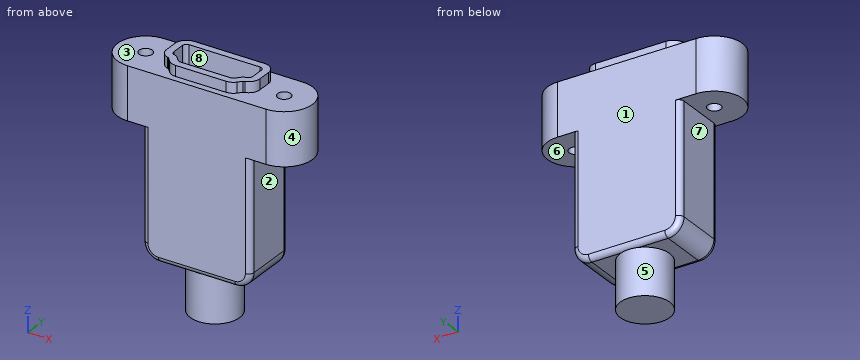
Autodesk Inventor part; units mm, degrees
ref_plane "YZ Plane" through (0, 0, 0) normal (1, 0, 0) x (0, 1, 0)
ref_plane "XZ Plane" through (0, 0, 0) normal (0, 1, 0) x (-1, 0, 0)
ref_plane "XY Plane" through (0, 0, 0) normal (0, 0, 1) x (1, 0, 0)
sketch "Sketch1" plane through (0, 0, 0) normal (0, 0, 1) x (1, 0, 0)
  line L0 (0, 0) -> (26.3, 0)
  line L1 (26.3, 10.7) -> (0, 10.7)
  arc A0 (0, 10.7) -> (0, 0) centre (0, 5.35) ccw
  arc A1 (26.3, 0) -> (26.3, 10.7) centre (26.3, 5.35) ccw
  circle A2 centre (0, 5.35) radius 1.25
  circle A3 centre (26.3, 5.35) radius 1.25
  dimension "d0" = 26.3
  dimension "d1" = 10.7
  dimension "d2" = 2.5
extrude "Extrusion1" add sketch "Sketch1" against normal blind 10
sketch "Sketch2" plane through (0, 0, 0) normal (0, 0, 1) x (1, 0, 0)
  line L0 (0, 0) -> (26.3, 0)
  arc A0 (0, 10.7) -> (0, 0) centre (0, 5.35) ccw
  line L1 (6.9455, 3.7725) -> (7.7604, 2.8465)
  line L2 (8.361, 2.575) -> (17.939, 2.575)
  line L3 (18.5396, 2.8465) -> (19.3545, 3.7725)
  line L4 (19.6057, 3.9348) -> (20.0852, 4.0824)
  line L5 (20.65, 4.847) -> (20.65, 7.325)
  line L6 (19.85, 8.125) -> (6.45, 8.125)
  line L7 (5.65, 7.325) -> (5.65, 4.847)
  line L8 (6.2148, 4.0824) -> (6.6943, 3.9348)
  line L9 (26.3, 10.7) -> (0, 10.7)
  arc A1 (6.45, 8.125) -> (5.65, 7.325) centre (6.45, 7.325) ccw
  arc A2 (20.65, 7.325) -> (19.85, 8.125) centre (19.85, 7.325) ccw
  arc A3 (5.65, 4.847) -> (6.2148, 4.0824) centre (6.45, 4.847) ccw
  arc A4 (20.0852, 4.0824) -> (20.65, 4.847) centre (19.85, 4.847) ccw
  arc A5 (6.9455, 3.7725) -> (6.6943, 3.9348) centre (6.5326, 3.4092) ccw
  arc A6 (19.6057, 3.9348) -> (19.3545, 3.7725) centre (19.7674, 3.4092) ccw
  arc A7 (7.7604, 2.8465) -> (8.361, 2.575) centre (8.361, 3.375) ccw
  arc A8 (17.939, 2.575) -> (18.5396, 2.8465) centre (17.939, 3.375) ccw
  line L10 (6.45, 9.4895) -> (19.85, 9.4895)
  arc A9 (22.0145, 7.325) -> (19.85, 9.4895) centre (19.85, 7.325) ccw
  line L11 (22.0145, 7.325) -> (22.0145, 4.847)
  arc A10 (20.4865, 2.7782) -> (22.0145, 4.847) centre (19.85, 4.847) ccw
  line L12 (20.4865, 2.7782) -> (20.2268, 2.6983)
  line L13 (20.2268, 2.6983) -> (19.5639, 1.945)
  arc A11 (17.939, 1.2105) -> (19.5639, 1.945) centre (17.939, 3.375) ccw
  line L14 (17.939, 1.2105) -> (8.361, 1.2105)
  arc A12 (6.7361, 1.945) -> (8.361, 1.2105) centre (8.361, 3.375) ccw
  line L15 (6.7361, 1.945) -> (6.0732, 2.6983)
  line L16 (6.0732, 2.6983) -> (5.8135, 2.7782)
  arc A13 (4.2855, 4.847) -> (5.8135, 2.7782) centre (6.45, 4.847) ccw
  line L17 (4.2855, 4.847) -> (4.2855, 7.325)
  arc A14 (6.45, 9.4895) -> (4.2855, 7.325) centre (6.45, 7.325) ccw
  point P0 (6.8428, 3.8892)
  point P1 (7.9994, 2.575)
  point P2 (18.3006, 2.575)
  point P3 (19.4572, 3.8892)
  point P4 (20.65, 4.2561)
  point P5 (20.65, 8.125)
  point P6 (5.65, 8.125)
  point P7 (5.65, 4.2561)
  dimension "d25" = 15
  dimension "d26" = 5.55
  dimension "d27" = 5.65
  dimension "d28" = 2.575
  dimension "d29" = 0.8
  dimension "d30" = 0.8
  dimension "d32" = 107.1
  dimension "d34" = 107.1
  dimension "d35" = 41.35
  dimension "d36" = 41.35
  dimension "d37" = 0.55
  dimension "d38" = 0.8
  dimension "d39" = 2.711
  dimension "d40" = 2.711
  dimension "d42" = 2.478
  dimension "d43" = 2.478
  dimension "d44" = 1.3645
extrude "Extrusion4" add sketch "Sketch2" along normal blind 2 contours A5 L8 A3 L7 A1 L6 A2 L5 A4 L4 A6 L3 A8 L2 A7 L1 | L10 A9 L11 A10 L12 L13 A11 L14 A12 L15 L16 A13 L17 A14
extrude "Extrusion5" cut sketch "Sketch2" against normal blind 4 and the other way blind 2 contours A5 L8 A3 L7 A1 L6 A2 L5 A4 L4 A6 L3 A8 L2 A7 L1
sketch "Sketch3" plane through (0, 0, -10) normal (0, 0, -1) x (-1, 0, 0)
  line L0 (-23.4, 0) -> (-2.9, 0)
  line L1 (-2.9, 0) -> (-2.9, 10.7)
  line L2 (-2.9, 10.7) -> (-23.4, 10.7)
  line L3 (-23.4, 10.7) -> (-23.4, 0)
  line L4 (0, 10.7) -> (-26.3, 10.7)
  arc A0 (-26.3, 10.7) -> (-26.3, 0) centre (-26.3, 5.35) ccw
  line L5 (-26.3, 0) -> (0, 0)
  dimension "d47" = 20.5
  dimension "d51" = 2.9
extrude "Extrusion6" add sketch "Sketch3" along normal blind 24 contours L3 L2 L1 L0
sketch "Sketch4" plane through (2.9, 10.7, -10) normal (0, 1, 0) x (-1, 0, 0)
  line L0 (-20.5, 0) -> (-20.5, -24)
  line L1 (-20.5, -24) -> (0, -24)
  arc A0 (-20.5, -21) -> (-17.5, -24) centre (-17.5, -21) ccw
  arc A1 (-3, -24) -> (0, -21) centre (-3, -21) ccw
  line L2 (-20.5, -21) -> (-20.5, -24)
  line L3 (-20.5, -24) -> (-17.5, -24)
  line L4 (-3, -24) -> (0, -24)
  line L5 (0, -24) -> (0, -21)
  line L6 (0, 0) -> (0, -24)
  point P0 (2.9, 10)
  dimension "d58" = 3
  dimension "d59" = 3
  dimension "d63" = 3
  dimension "d64" = 3
  dimension "d65" = 3
  dimension "d66" = 3
extrude "Extrusion7" cut sketch "Sketch4" against normal through all
fillet "Fillet1" radius 1 10 edges at (22.5213, 10.7, -33.1213) (13.15, 10.7, -34) (3.7787, 10.7, -33.1213) (2.9, 10.7, -20.5) (23.4, 10.7, -20.5) (22.5213, 0, -33.1213) (13.15, 0, -34) (3.7787, 0, -33.1213) (2.9, 0, -20.5) (23.4, 0, -20.5)
sketch "Sketch5" plane through (0, 0, -34) normal (0, 0, -1) x (-1, 0, 0)
  circle A0 centre (-13.15, 5.35) radius 4.7
  line L0 (-5.9, 10.7) -> (-20.4, 10.7)
  line L1 (-23.4, 1) -> (-23.4, 9.7)
  point P0 (0, 0)
  dimension "d67" = 9.4
  dimension "d68" = 5.35
  dimension "d69" = 10.25
extrude "Extrusion8" add sketch "Sketch5" along normal blind 8.8
equation "\"d27\" = -0.5 * d25 + 0.5 * d0"
equation "\"d28\" = -0.5 * d26 + 0.5 * d1"
equation "\"d34\" = d32"
equation "\"d36\" = d35"
equation "\"d40\" = d39"
equation "\"d43\" = d42"
equation "\"d51\" = -0.5 * d47 + 0.5 * d0"
equation "\"d58\" = d54"
equation "\"d59\" = d54"
equation "\"d63\" = d54"
equation "\"d64\" = d54"
equation "\"d65\" = d54"
equation "\"d66\" = d54"
equation "\"d68\" = 0.5 * d1"
equation "\"d69\" = 0.5 * d47"
properties part number "hdmi-panel-mount"
CAD build for the part. Positions are in the model's coordinates, mm. Face numbers are marked on the shaded views. A direction names the side the tool comes from. Round coordinates to 2 decimals unless told otherwise and drop trailing zeros. Order: outer loops, then holes, each group sorted by start corner. A loop starts at its lowest first (then second) coordinate and runs counter-clockwise, first axis right, second up. Notation, with made-up numbers: (-27, 34) -> (-14, 34) arc R22 cw to (-14, 45) -> close; hole circle Ø7 at (38.25, -2.75). An arc over 180 degrees is marked (long way). One line per question, with ' | ' between items.
Q1. Probe probe 1 along X at (y, z) = (5.75, -2.5); probe 2 along Y at (x, z) = (0, -7); probe 3 along Z at (x, y) = (19.5, 5.25). List the from-to ranges inside material, lowest first.
Completed:
probe 1: x = -5.34 to -1.18, 1.18 to 5.65, 20.65 to 25.12, 27.48 to 31.64 | probe 2: y = 0 to 4.1, 6.6 to 10.7 | probe 3: z = -34 to -4
Q2. Slice it at D-D (z = -6.5). Write the cut outline in (x, y), then the cut area to 3 significant figures.
Completed:
outline: (0, 0) -> (26.3, 0) arc R5.35 ccw to (26.3, 10.7) -> (0, 10.7) arc R5.35 ccw to start; hole circle Ø2.5 at (0, 5.35); hole circle Ø2.5 at (26.3, 5.35) | area: 362 mm^2
Q3. Two-plate mould, pull along X, no slides. Class the marked faces 6, 7 and 8: released by +X, released by -X, zero draft, split by the parting line, or undercut.
Completed:
face 6: zero draft | face 7: released by -X | face 8: undercut
Q4. Drop flat-ended pins along their axis: pin 1 (2.5 mm diameter, centred on y = 5, z = -25, fed in from -X); pin 2 (2.5 mm diameter, centred on y = 6.5, z = -17.5, fed in from +X); pin 3 (1 mm diameter, centred on x = -1, y = 7, fed in from -Z). Give the stop position or say it passes through.
Completed:
pin 1: stops at x = 2.9 | pin 2: stops at x = 23.4 | pin 3: stops at z = -10
Q5. Slice it at A-A (y = 5.35). Give the number of separate pieces and of enclosed holes in the cut face, then the cut area to 3 significant figures.
Completed:
separate pieces: 3 | enclosed holes: 0 | area: 836 mm^2
Q6. Which spindle directions (+Z, -Z, +X, -X, +Y, -Y) get a long thin tool onto all of the face, cutting with end or side? Do the marked faces 1, 2, 3, 4 and 5. Say none if no direction does.
Completed:
face 1: +Z, -Z, +X, -X, +Y | face 2: -Z, +X, +Y, -Y | face 3: +Z | face 4: +Z, -Z, +X | face 5: -Z
